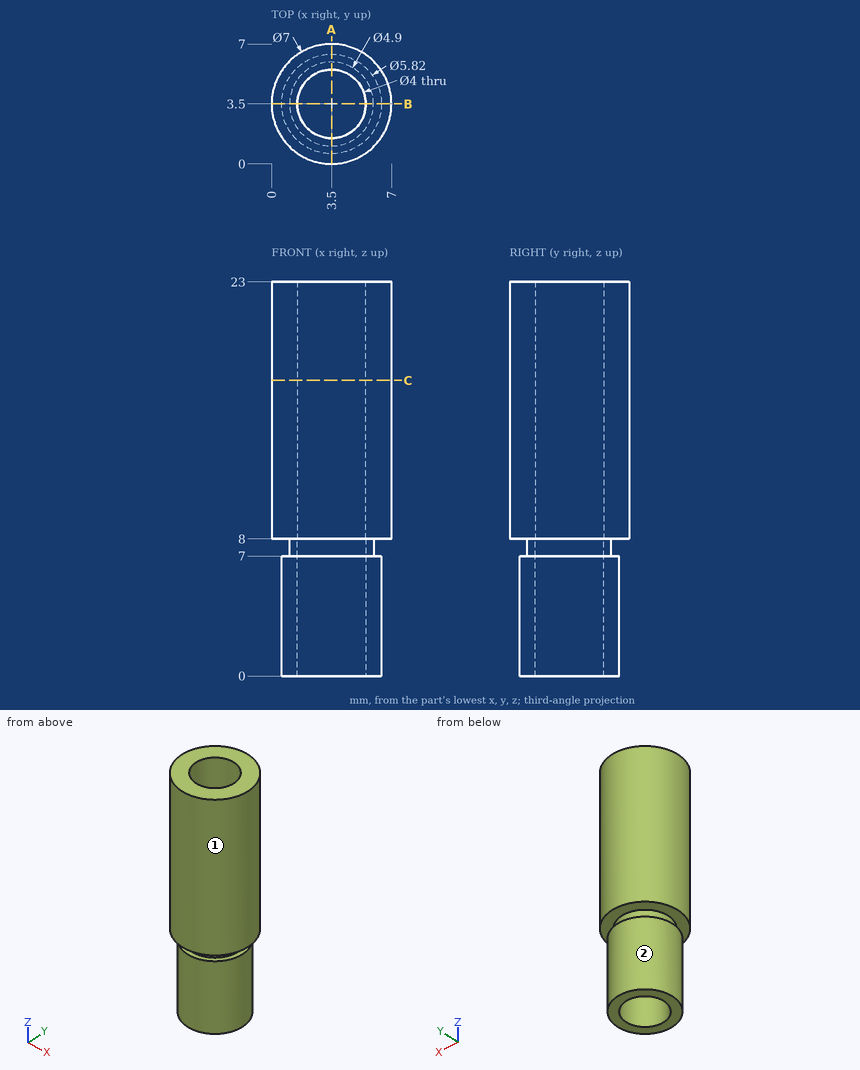
Check sheet for the drawn part. Datum: minimum x, y, z corner. Units: mm. A direction names the side the tool comes from. Round coordinates to 2 decimals unless told otherwise and drop trailing zeros. Order: outer loops, then holes, each group sorted by start corner. A loop starts at its lowest first (then second) coordinate and runs counter-clockwise, first axis right, second up. Notation, with made-up numbers: (76.5, 12) - (130.5, 12) arc R22 cw to (130.5, 25) - close; hole circle Ø10 at (29.25, 81.5). An arc over 180 degrees is marked (long way). Use a Markdown table: item, result. Add a question column.
(1) Tool access check on the marked faces 1 and 2. Record the directions out of +Z, -Z, +X, -X, +Y, -Y that give a thin tool (end or side, any length) a straight path to the whole face; none if there is none.
(2) Sectioned sample at C-C, the plane z = 17.25. Enter the section's corners in (x, y).
(3) Depth check by flat-ended pin: pin 1 (2 mm diameter, centred on x = 4.5, y = 4.5, fed in from -Z); pin 2 (2 mm diameter, centred on y = 1, z = 16.5, fed in from +X). Enter the tip coordinate at first touch or a pass-through.
(4) Sectioned sample at A-A, the plane x = 3.5. Enter the section's corners in (y, z).
(5) Material ranges on line 1 along X through (y, z) = (3.5, 3.25); line 2 along Y through (x, z) = (3.5, 18.75), recorded low to high. Write a range as [from, to].
Answers below:
| question | item | result |
|---|---|---|
| 1 | face 1 | +Z, -Z |
| 1 | face 2 | -Z |
| 2 | outline | circle Ø7 at (3.5, 3.5); hole circle Ø4 at (3.5, 3.5) |
| 3 | pin 1 | z = 0 |
| 3 | pin 2 | x = 6.66 |
| 4 | outline | (0, 8) - (1.05, 8) - (1.05, 7) - (0.59, 7) - (0.59, 0) - (1.5, 0) - (1.5, 23) - (0, 23) - close; (5.5, 0) - (6.41, 0) - (6.41, 7) - (5.95, 7) - (5.95, 8) - (7, 8) - (7, 23) - (5.5, 23) - close |
| 5 | line 1 | [0.59, 1.5], [5.5, 6.41] |
| 5 | line 2 | [0, 1.5], [5.5, 7] |
